Autodesk Inventor part; units mm, degrees
ref_plane "YZ Plane" through (0, 0, 0) normal (1, 0, 0) x (0, 1, 0)
ref_plane "XZ Plane" through (0, 0, 0) normal (0, 1, 0) x (-1, 0, 0)
ref_plane "XY Plane" through (0, 0, 0) normal (0, 0, 1) x (1, 0, 0)
sketch "Sketch1" plane through (0, 0, 0) normal (0, 1, 0) x (-1, 0, 0)
  point P0 (0, 0)
sketch "Sketch2" plane through (0, 0, 0) normal (0, 1, 0) x (-1, 0, 0)
  line L0 (0, -4.7625) -> (0, -37.4015)
  line L1 (4.7625, -42.164) -> (58.7375, -42.164)
  line L2 (63.5, -37.4015) -> (63.5, -4.7625)
  line L3 (58.7375, 0) -> (4.7625, 0)
  arc A0 (4.7625, 0) -> (0, -4.7625) centre (4.7625, -4.7625) ccw
  circle A1 centre (4.7625, -4.7625) radius 4.7625
  circle A2 centre (4.7625, -4.7625) radius 2.3813
  arc A3 (0, -37.4015) -> (4.7625, -42.164) centre (4.7625, -37.4015) ccw
  arc A4 (58.7375, -42.164) -> (63.5, -37.4015) centre (58.7375, -37.4015) ccw
  arc A5 (63.5, -4.7625) -> (58.7375, 0) centre (58.7375, -4.7625) ccw
  circle A6 centre (58.7375, -4.7625) radius 4.7625
  circle A7 centre (58.7375, -37.4015) radius 4.7625
  circle A8 centre (58.7375, -4.7625) radius 2.3813
  circle A9 centre (58.7375, -37.4015) radius 2.3813
  point P0 (0, 0)
  point P1 (0, -42.164)
  point P2 (63.5, -42.164)
  point P3 (4.7625, 0)
  point P4 (4.7625, 0)
  dimension "d0" = 42.164
  dimension "d1" = 63.5
  dimension "d2" = 4.7625
  dimension "d3" = 4.7625
  dimension "d4" = 4.7625
  dimension "d5" = 4.7625
  dimension "d6" = 4.7625
extrude "Extrusion1" add sketch "Sketch2" along normal blind 9.525 contours A0 A1 | A5 A6 | A7 A4
extrude "Extrusion2" add sketch "Sketch2" along normal blind 4.7625 contours A1 L3 A6 L2 A7 L1 A3 L0
sketch "Sketch3" plane through (0, 4.7625, 0) normal (0, 1, 0) x (1, 0, 0)
  circle A0 centre (-4.7625, 4.7625) radius 2.3813
  line L0 (-4.7625, 4.7625) -> (-1.3949, 1.3949)
  circle A1 centre (-4.7625, 4.7625) radius 4.7625
  line L1 (-4.7625, 4.7625) -> (0, 4.7625) construction
  circle A2 centre (-4.7625, 4.7625) radius 4.7625
  circle A3 centre (-4.7625, 4.7625) radius 2.3813
  circle A4 centre (-58.7375, 4.7625) radius 4.7625
  circle A5 centre (-58.7375, 4.7625) radius 4.7625
  circle A6 centre (-58.7375, 4.7625) radius 2.3813
  circle A7 centre (-58.7375, 37.4015) radius 2.3813
  circle A8 centre (-58.7375, 37.4015) radius 4.7625
  circle A9 centre (-58.7375, 37.4015) radius 2.3813
  circle A10 centre (-58.7375, 37.4015) radius 2.3813
  point P0 (0, 0)
  dimension "d22" = 45
extrude "Extrusion3" add sketch "Sketch3" along normal blind 20.0025
sketch "Sketch4" plane through (0, 4.7625, 0) normal (0, 1, 0) x (1, 0, 0)
  line L0 (0, 4.7625) -> (0, 37.4015)
  line L1 (0, 21.082) -> (0, 26.797)
  line L2 (0, 26.797) -> (0, 21.082)
  line L3 (0, 21.082) -> (0, 15.367)
  line L4 (0, 15.367) -> (7.62, 15.367)
  line L5 (7.62, 15.367) -> (7.62, 26.797)
  line L6 (7.62, 26.797) -> (0, 26.797)
  line L7 (7.62, 26.797) -> (0, 34.417)
  line L8 (7.62, 26.797) -> (18.3963, 26.797) construction
  line L9 (7.62, 15.367) -> (0, 7.747)
  line L10 (7.62, 15.367) -> (18.3963, 15.367) construction
  point P0 (0, 0)
  dimension "d25" = 5.715
  dimension "d26" = 5.715
  dimension "d27" = 7.62
  dimension "d28" = 135
  dimension "d29" = 135
extrude "Extrusion4" add sketch "Sketch4" against normal blind 4.7625
sketch "Sketch5" plane through (0, 4.7625, 0) normal (0, 1, 0) x (1, 0, 0)
  line L0 (7.62, 26.797) -> (7.62, 15.367)
  line L1 (7.62, 15.367) -> (-6.35, 15.367)
  line L2 (-6.35, 15.367) -> (-6.35, 26.797)
  line L3 (-6.35, 26.797) -> (7.62, 26.797)
  line L4 (0, 7.747) -> (7.62, 15.367)
  line L5 (7.62, 15.367) -> (7.62, 26.797)
  line L6 (7.62, 15.367) -> (7.62, 26.797)
  point P0 (0, 0)
  dimension "d32" = 13.97
sketch "Sketch6" plane through (0, 4.7625, 0) normal (0, 1, 0) x (1, 0, 0)
  point P0 (0, 0)
extrude "Extrusion5" add sketch "Sketch5" along normal blind 9.525
sketch "Sketch7" plane through (7.62, 0, -15.367) normal (1, 0, 0) x (0, 0, -1)
  line L0 (0, 4.7625) -> (11.43, 4.7625)
  line L1 (5.715, 4.7625) -> (5.715, 17.145)
  circle A0 centre (5.715, 17.145) radius 5.715
  point P0 (-15.367, 0)
  dimension "d35" = 12.3825
  dimension "d36" = 11.43
extrude "Extrusion6" cut sketch "Sketch7" against normal blind 9.9441
sketch "Sketch8" plane through (0, 4.7625, 0) normal (0, 1, 0) x (1, 0, 0)
  line L0 (-58.7375, 0) -> (-4.7625, 0)
  line L1 (-31.75, 0) -> (-31.75, 42.164)
  line L2 (-4.7625, 42.164) -> (-58.7375, 42.164)
  circle A0 centre (-31.75, 21.082) radius 2.3812
  point P0 (0, 0)
  dimension "d39" = 4.7625
extrude "Extrusion7" cut sketch "Sketch8" against normal blind 9.9441
sketch "Sketch9" plane through (0, 0, 0) normal (0, -1, 0) x (1, 0, 0)
  arc A0 (-4.7625, -42.164) -> (0, -37.4015) centre (-4.7625, -37.4015) ccw
  circle A1 centre (-4.7625, -37.4015) radius 2.3813
  circle A2 centre (-4.7625, -4.7625) radius 2.3813
  point P0 (0, 0)
extrude "Extrusion8" cut sketch "Sketch9" against normal up to surface (4.7625 mm away) contours A1
sketch "Sketch10" plane through (0, 4.7625, 0) normal (0, 1, 0) x (1, 0, 0)
  circle A0 centre (-4.7625, 37.4015) radius 2.3813
  circle A1 centre (-4.7625, 37.4015) radius 4.7625
  point P0 (0, 0)
extrude "Extrusion9" add sketch "Sketch10" along normal up to surface (20.0025 mm away)
sketch "Sketch11" plane through (0, 4.7625, 0) normal (0, 1, 0) x (1, 0, 0)
  circle A0 centre (-31.75, 21.082) radius 2.3812
  circle A1 centre (-31.75, 21.082) radius 2.3812
  point P0 (0, 0)
extrude "Extrusion10" add sketch "Sketch11" against normal up to surface (4.7625 mm away)
sketch "Sketch12" plane through (-2.3241, 0, -15.367) normal (1, 0, 0) x (0, 0, -1)
  arc A0 (0.7657, 14.2875) -> (10.6643, 14.2875) centre (5.715, 17.145) ccw
  circle A1 centre (5.715, 17.145) radius 5.715
  line L0 (0.7657, 14.2875) -> (10.6643, 14.2875)
  line L1 (11.43, 14.2875) -> (0, 14.2875)
  point P0 (-15.367, 0)
extrude "Extrusion11" add sketch "Sketch12" along normal up to surface (9.9441 mm away) contours L0 A0
sketch "Sketch13" plane through (0, 0, 0) normal (0, -1, 0) x (1, 0, 0)
  arc A0 (-58.7375, 0) -> (-63.5, -4.7625) centre (-58.7375, -4.7625) ccw
  line L0 (-63.5, -4.7625) -> (-63.5, 0)
  line L1 (-63.5, 0) -> (-63.5, 3.81)
  circle A1 centre (-58.7375, 8.5725) radius 4.7625
  arc A2 (-63.5, -4.7625) -> (-58.7375, 0) centre (-58.7375, -4.7625) ccw
  line L2 (-63.5, 3.81) -> (-53.975, 3.81)
  line L3 (-53.975, 3.81) -> (-53.975, 0)
  line L4 (-58.7375, 0) -> (-4.7625, 0)
  line L5 (-63.5, 8.5725) -> (-63.5, 3.81)
  circle A3 centre (-58.7375, 8.5725) radius 2.3813
  circle A4 centre (-58.7375, -4.7625) radius 2.3813
  line L6 (-53.975, 8.5725) -> (-53.975, 3.81)
  circle A5 centre (-4.7625, 8.5725) radius 2.3813
  circle A6 centre (-4.7625, 8.5725) radius 4.7625
  circle A7 centre (-4.7625, -4.7625) radius 2.3813
  arc A8 (0, -4.7625) -> (-4.7625, 0) centre (-4.7625, -4.7625) ccw
  line L7 (0, -4.7625) -> (0, 8.5725)
  line L8 (-9.525, 8.5725) -> (-9.525, 0)
  circle A9 centre (-58.7375, -50.7365) radius 2.3813
  circle A10 centre (-58.7375, -50.7365) radius 4.7625
  circle A11 centre (-58.7375, -37.4015) radius 2.3813
  arc A12 (-63.5, -37.4015) -> (-58.7375, -42.164) centre (-58.7375, -37.4015) ccw
  line L9 (-63.5, -37.4015) -> (-63.5, -50.7365)
  line L10 (-63.5, -37.4015) -> (-63.5, -4.7625)
  line L11 (-53.975, -50.7365) -> (-53.975, -42.164)
  line L12 (-4.7625, -42.164) -> (-58.7375, -42.164)
  circle A13 centre (-4.7625, -50.7365) radius 2.3813
  circle A14 centre (-4.7625, -50.7365) radius 4.7625
  circle A15 centre (-4.7625, -37.4015) radius 2.3813
  arc A16 (-4.7625, -42.164) -> (0, -37.4015) centre (-4.7625, -37.4015) ccw
  line L13 (0, -37.4015) -> (0, -50.7365)
  line L14 (0, -34.417) -> (0, -37.4015)
  line L15 (-9.525, -50.7365) -> (-9.525, -42.164)
  point P0 (0, 0)
  point P1 (0, -50.7365)
  point P2 (0, 8.5725)
  dimension "d50" = 3.81
  dimension "d51" = 9.525
  dimension "d52" = 13.335
  dimension "d53" = 13.335
  dimension "d54" = 13.335
  dimension "d55" = 13.335
extrude "Extrusion12" add sketch "Sketch13" against normal up to surface (4.7625 mm away) contours A0 L0 L1 L2 L3 L4 | L2 A1 L6 | L5 A1 L2 | A1 | L8 A6 L7 A8 L4 | A6 | A10 | A10 L9 A12 L12 L11 | A16 L13 A14 L15 L12 | A14
properties part number "MotorBot_3DPrint"
Here's how the part is built. I have some questions about the finished solid (model axes, mm). A direction names the side the tool comes from. Coordinates: 2 decimals unless noted, no trailing zeros. Order: outer loops, then holes, each group sorted by start corner. A loop starts at its lowest first (then second) coordinate and runs counter-clockwise, first axis right, second up.
1) Which directions (+Z, -Z, +X, -X, +Y, -Y) give clear straight access to the entire face, cutting with the end or side of a thin tool? Please do faces 1 (the face through (0, 2, 1)), 2 (the face through (1, 14.288, -21)), 3 (the face through (-9.525, 2, 4)), 4 (the face through (-53.975, 2, -47)), 5 (the face through (-4.45, 14.62, -0.01)).
2) Imagine slicing it at C-C on y = 2.5. State how many separate pieces and enclosed holes the cut face has, and give its area (3 significant figures).
3) Imagine slicing it at B-B on y = 16. List the corners of the cut face in (x, z) for me (1 decimal), and give its area (3 significant figures).
4) I need wall thicknesses on line 1 (Z direction, x = -57, y = 11.5); line 2 (Z direction, x = -3, y = 12.75); line 3 (Z direction, x = -57.5, y = 6.75). Which ranges of each line are inside material? Lowest first, please.
5) Will these pins go through, and if not, where does the flat tip stop? pin 1 (4 mm diameter, centred on y = 3.5, z = -43, fed in from +X); pin 2 (5 mm diameter, centred on y = 7.5, z = -21.5, fed in from -X); pin 3 (5 mm diameter, centred on x = -29, y = 2.5, fed in from -Z).
6) We'd pull the mould along Z, two halves only. Please class faces 6 (the face through (-56.466, 2.348, 9.288)), 7 (the face through (-5.279, 12.209, -39.726)), 8 (the face through (-4, 24.765, -40)), 9 (the face through (-58.8, 2.3, -55.5)): +Z half, -Z half, draft (parallel to the pull), parting line (faces both ways), or undercut.
7) Imagine slicing it at A-A on z = 3. List the corners of the cut face in (x, y) for me (1 decimal), and give its area (3 significant figures).
8) Imagine slicing it at D-D on z = -19. List the corners of the cut face in (x, y) for me, and give its area (3 significant figures).
Response values:
1. face 1: +Z, +X, +Y, -Y
1. face 2: +X, -X, +Y
1. face 3: +Z, +Y, -Y
1. face 4: -Z, +Y, -Y
1. face 5: +Y
2. separate pieces: 1
2. enclosed holes: 8
2. area: 3,150 mm2
3. outline: circle Ø9.5 at (-58.7, -37.4); circle Ø9.5 at (-58.7, -4.8); circle Ø9.5 at (-4.8, -37.4); circle Ø9.5 at (-4.8, -4.8); hole circle Ø4.8 at (-58.7, -37.4); hole circle Ø4.8 at (-58.7, -4.8); hole circle Ø4.8 at (-4.8, -37.4); hole circle Ø4.8 at (-4.8, -4.8)
3. area: 214 mm2
4. line 1: z = -41.84 to -39.03, -35.77 to -32.97, -9.2 to -6.39, -3.13 to -0.33
4. line 2: z = -41.83 to -39, -35.8 to -32.98, -26.8 to -15.37, -9.19 to -6.36, -3.16 to -0.34
4. line 3: z = -42 to -39.44, -35.37 to -32.8, -9.36 to -6.8, -2.73 to -0.16
5. pin 1: stops at x = 0
5. pin 2: stops at x = -6.35
5. pin 3: stops at z = -42.16
6. face 6: undercut
6. face 7: undercut
6. face 8: draft
6. face 9: -Z half
7. outline: (-63.5, 0) - (-54, 0) - (-54, 4.8) - (-63.5, 4.8) - close; (-9.5, 0) - (0, 0) - (0, 4.8) - (-9.5, 4.8) - close
7. area: 90.7 mm2
8. outline: (-63.5, 0) - (7.62, 0) - (7.62, 14.29) - (-6.35, 14.29) - (-6.35, 4.76) - (-63.5, 4.76) - close
8. area: 472 mm2
